Part model, mm, in its own coordinate system. Face numbers are marked on the shaded views. Give positions to 0.01 mm unless a question says otherwise; leave off trailing zeros. Order: outer loops, then holes, each group sorted by start corner. A loop starts at its lowest first (then second) coordinate and runs counter-clockwise, first axis right, second up. Notation, with made-up numbers: (53.5, 16.25) -> (64.5, 16.25) arc R16 cw to (64.5, 46.25) -> close; hole circle Ø10 at (-30.75, 7.5). An arc over 180 degrees is marked (long way). Write item = value, one per line. Start each with the question number.
(1) Probe line 1 along Y through (x, z) = (-0.25, -3.9); line 2 along Z through (x, y) = (-5.75, -5.5). List the from-to ranges inside material, lowest first. Write a range as from..to.
(2) Saw through at C-C, the plane z = -2.55. List the corners of the cut face in (x, y), then the cut area to 3 significant figures.
(3) Flat gauge pins, fed straight in: pin 1 (13.5 mm diameter, centred on x = 0, y = 3, fed in from -Z); pin 2 (4 mm diameter, centred on x = 4.5, y = 0, fed in from -Z); pin 3 (2 mm diameter, centred on x = -6.5, z = -1.5, fed in from -Y); pin 4 (7.5 mm diameter, centred on x = 0, y = 0, fed in from -Z). Where does each tip first touch, or does it go through?
(4) Two-plate mould, pull along Y, no slides. Class the marked faces 1, 2 and 3: pulls with the +Y half, pulls with the -Y half, needs draft (parallel to the pull), parting line crosses it, or undercut.
(5) Saw through at A-A, the plane y = 0. List the corners of the cut face in (x, z).
from build123d import *

# Parameters (mm, degrees)
F2_T     = -0.65
F3_R     = 4.8
F4_DEPTH = 4.601


with BuildPart() as f1:
    # F0 (on Front) → F1 (revolve)
    with BuildSketch(Plane.XZ):
        with BuildLine():
            Line((8.5, 0), (0, 0))
            Line((0, 0), (0, -4.6))
            Line((0, -4.6), (11.5, -4.6))
            Line((11.5, -4.6), (11.5, -3))
            ThreePointArc((11.5, -3), (10.62132, -0.87868), (8.5, 0))
        make_face()
    revolve(axis=Axis((0, 0, -2.3), (0, 0, -1)))

    # F2
    f2_openings = [f1.faces().sort_by_distance(p)[0] for p in [
        (0, 0, -4.6),
    ]]
    offset(amount=F2_T, openings=f2_openings)

    # F3 (on face) → F4 (cut, through all)
    with BuildSketch(Plane.XY):
        Circle(F3_R)
    extrude(amount=-F4_DEPTH, mode=Mode.SUBTRACT)


solid = f1.part
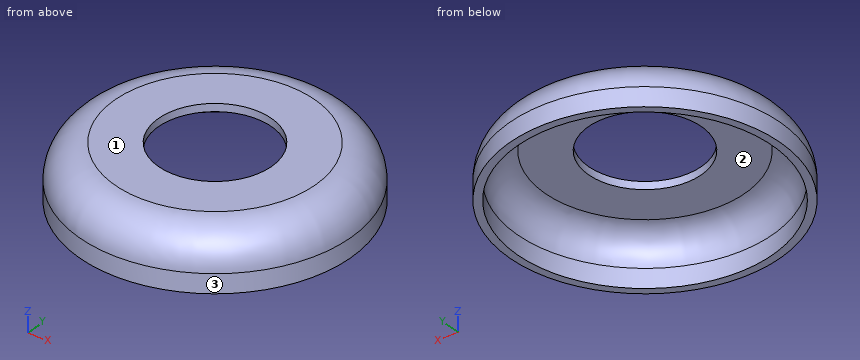
Results list:
q1.line_1 = -11.5..-10.85, 10.85..11.5
q1.line_2 = -0.65..0
q2.outline = circle Ø22.93 at (0, 0); hole circle Ø21.61 at (0, 0)
q2.area = 46.1 mm^2
q3.pin_1 = -1.01
q3.pin_2 = -0.65
q3.pin_3 = -9.83
q3.pin_4 = through
q4.face_1 = needs draft
q4.face_2 = undercut
q4.face_3 = parting line crosses it
q5.outline = (-11.5, -4.6) -> (-10.85, -4.6) -> (-10.85, -3) arc R2.35 cw to (-8.5, -0.65) -> (-4.8, -0.65) -> (-4.8, 0) -> (-8.5, 0) arc R3 ccw to (-11.5, -3) -> close; (4.8, -0.65) -> (8.5, -0.65) arc R2.35 cw to (10.85, -3) -> (10.85, -4.6) -> (11.5, -4.6) -> (11.5, -3) arc R3 ccw to (8.5, 0) -> (4.8, 0) -> close
